Can you work these out from the drawing? Everything is in mm from the part's minimum corner. Give positions to 0.01 mm unless a question says otherwise; leave off trailing zeros. Loops run counter-clockwise (first coordinate to the right, second up) from the corner with the lowest first, then second, coordinate; pieces in that order, holes last. Notation, with made-up numbers: (25.5, 0.25) - (74.5, 0.25) arc R21 cw to (74.5, 39.25) - close; hole circle Ø1 at (33.25, 0). An arc over 180 degrees is marked (long way). Answer in a Markdown table with one row per item.
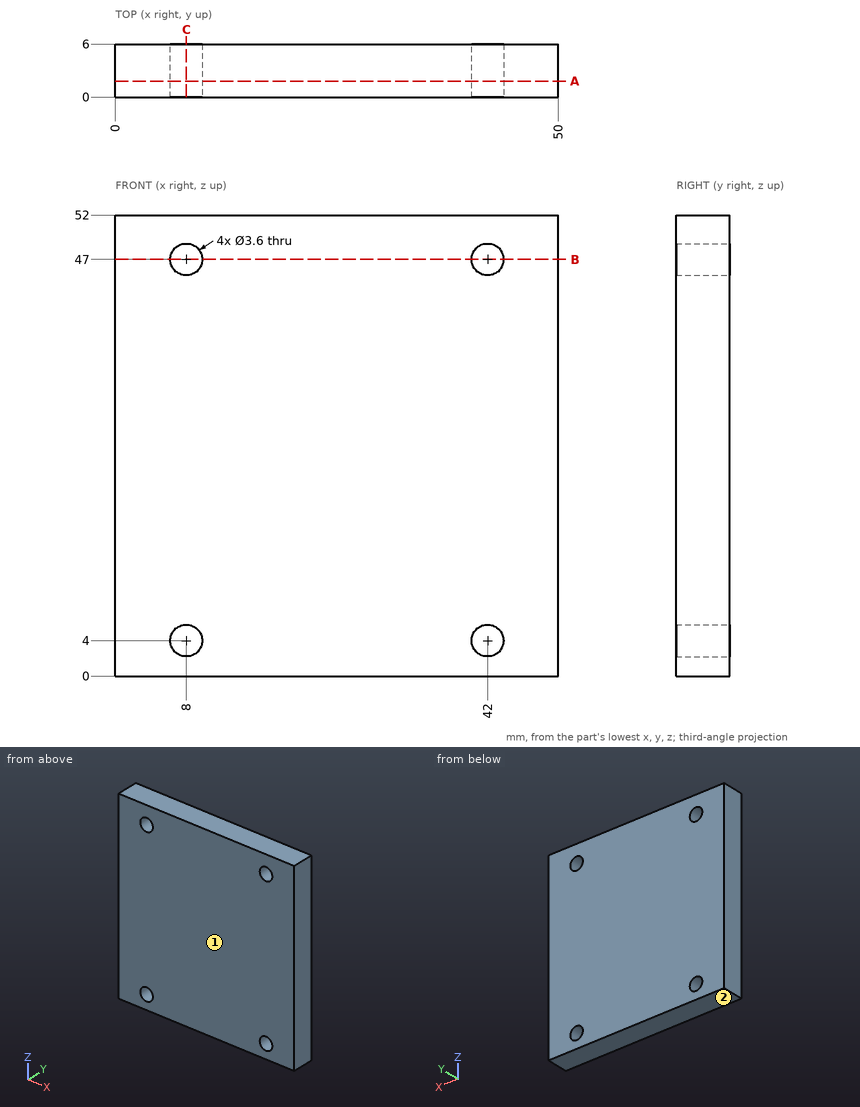
Q1. Imagine slicing it at C-C, the plane x = 8. Write out the boundary of the cut face in (y, z), and give its area (3 significant figures).
Checked values:
| item | result |
|---|---|
| outline | (0, 0) - (6, 0) - (6, 2.2) - (0, 2.2) - close; (0, 5.8) - (6, 5.8) - (6, 45.2) - (0, 45.2) - close; (0, 48.8) - (6, 48.8) - (6, 52) - (0, 52) - close |
| area | 269 mm² |
Q2. If we mould it in two halves opening along Z, with no side actions, what happens to the marked faces 1 and 2? For each: released by +Z, released by -Z, zero draft, split by the parting line, or undercut.
Checked values:
| item | result |
|---|---|
| face 1 | zero draft |
| face 2 | released by -Z |
Q3. Imagine slicing it at B-B, the plane z = 47. Write out the boundary of the cut face in (x, y).
Checked values:
| item | result |
|---|---|
| outline | (0, 0) - (6.2, 0) - (6.2, 6) - (0, 6) - close; (9.8, 0) - (40.2, 0) - (40.2, 6) - (9.8, 6) - close; (43.8, 0) - (50, 0) - (50, 6) - (43.8, 6) - close |
Q4. For pin 1 (6 mm diameter, centred on x = 42, z = 4, fed in from +Y), with a flat end and sliding along its axis, tell me the tip position at first contact or that it passes through.
Checked values:
| item | result |
|---|---|
| pin 1 | stops at y = 6 |
Q5. If I drill on line 1 (Z direction, x = 42, y = 1.65); line 2 (X direction, y = 3.9, z = 4); line 3 (Z direction, x = 41, y = 5.25), over which ranges is the centre line in solid material (lowest first)? Write a range as [from, to].
Checked values:
| item | result |
|---|---|
| line 1 | z = [0, 2.2], [5.8, 45.2], [48.8, 52] |
| line 2 | x = [0, 6.2], [9.8, 40.2], [43.8, 50] |
| line 3 | z = [0, 2.5], [5.5, 45.5], [48.5, 52] |
Q6. Imagine slicing it at A-A, the plane y = 1.8. Write out the boundary of the cut face in (x, z).
Checked values:
| item | result |
|---|---|
| outline | (0, 0) - (50, 0) - (50, 52) - (0, 52) - close; hole circle Ø3.6 at (8, 4); hole circle Ø3.6 at (8, 47); hole circle Ø3.6 at (42, 4); hole circle Ø3.6 at (42, 47) |
